Could you check a few things on this model? Use its own coordinates, in mm. A direction names the side the tool comes from. Round coordinates to 2 decimals unless told otherwise and drop trailing zeros. Loops run counter-clockwise (first coordinate to the right, second up) from the corner with the lowest first, then second, coordinate; pieces in that order, holes last. Notation, with made-up numbers: (48.25, -24.75) -> (100.25, -24.75) arc R24 ccw to (100.25, -11.75) -> close; hole circle Ø5 at (62, -23.5). An arc over 180 degrees is marked (long way). One line per item, written item: value.
Autodesk Inventor part; units mm, degrees
ref_plane "РабПлоскость1" through (0, 14.5, 0) normal (0, 1, 0) x (-1, 0, 0)
ref_plane "РабПлоскость2" through (0, 0, 18.5) normal (0, 0, 1) x (1, 0, 0)
ref_plane "YZ Plane" through (0, 0, 0) normal (1, 0, 0) x (0, 1, 0)
sketch "Эскиз1" plane through (0, 0, 0) normal (0, 0, 1) x (1, 0, 0)
  line L0 (0, 0) -> (-160, 0)
  line L1 (0, 0) -> (0, 15.4226)
  line L2 (0, 15.4226) -> (-1, 16)
  line L3 (-1, 16) -> (-60, 16)
  line L4 (-60, 16) -> (-60, 17.5)
  line L5 (-60, 17.5) -> (-80, 17.5)
  line L6 (-80, 17.5) -> (-80, 20)
  line L7 (-80, 20) -> (-140, 20)
  line L8 (-140, 20) -> (-140, 17.5)
  line L9 (-140, 17.5) -> (-160, 17.5)
  line L10 (-160, 17.5) -> (-160, 0)
  dimension "d0" = 160
  dimension "d1" = 32
  dimension "d2" = 30
  dimension "d3" = 1
  dimension "d4" = 60
  dimension "d5" = 35
  dimension "d6" = 20
  dimension "d7" = 40
revolve "Вращение1" add sketch "Эскиз1" angle 360 about axis through (0, 0, 0) along (-1, 0, 0)
ref_plane "РабПлоскость1" through (0, 14.5, 0) normal (0, 1, 0) x (-1, 0, 0)
ref_plane "РабПлоскость2" through (0, 0, 18.5) normal (0, 0, 1) x (1, 0, 0)
sketch "Эскиз3" plane through (0, 14.5, 0) normal (0, 1, 0) x (-1, 0, 0)
  line L0 (0, 15.4226) -> (0, -15.4226)
  line L1 (80, 20) -> (80, -20)
  line L2 (140, 20) -> (140, -20)
  line L3 (44, 0) -> (16, 0) construction
  line L4 (40, 4) -> (20, 4)
  line L5 (20, -4) -> (40, -4)
  arc A0 (40, -4) -> (40, 4) centre (40, 0) ccw
  arc A1 (20, 4) -> (20, -4) centre (20, 0) ccw
  point P0 (0, 0)
  point P1 (30, 0)
  point P2 (80, 0)
  dimension "d11" = 20
  dimension "d12" = 8
  dimension "d13" = 50
extrude "Выдавливание1" cut sketch "Эскиз3" along normal through all
sketch "Эскиз4" plane through (0, 0, 18.5) normal (0, 0, 1) x (1, 0, 0)
  line L0 (-124, 0) -> (-96, 0) construction
  line L1 (-120, -4) -> (-100, -4)
  line L2 (-100, 4) -> (-120, 4)
  arc A0 (-120, 4) -> (-120, -4) centre (-120, 0) ccw
  arc A1 (-100, -4) -> (-100, 4) centre (-100, 0) ccw
  line L3 (-80, -17.5) -> (-80, 17.5)
  point P0 (0, 0)
  point P1 (-110, 0)
  point P2 (-80, 0)
  dimension "d16" = 20
  dimension "d17" = 8
  dimension "d18" = 30
extrude "Выдавливание2" cut sketch "Эскиз4" along normal through all
properties part number "Shaft1"
Item 1: For faces 1 (the face through (-30.91, -3.47, 15.62)), 2 (the face through (-16, 15, 0)), 3 (the face through (-110, 0, 18.5)), 4 (the face through (-140, 0, 18)), which set-ups out of +Z, -Z, +X, -X, +Y, -Y let a thin tool reach every point of the face, with its end or its side?
Output:
face 1: +X
face 2: +Y
face 3: +Z
face 4: -X
Item 2: If we section it at A-A on z = 0: List the corners of the cut face in (x, y) for me, plus the area to 3 significant figures.
Output:
outline: (-160, -17.5) -> (-140, -17.5) -> (-140, -20) -> (-80, -20) -> (-80, -17.5) -> (-60, -17.5) -> (-60, -16) -> (-1, -16) -> (0, -15.42) -> (0, 15.42) -> (-1, 16) -> (-16, 16) -> (-16, 14.5) -> (-44, 14.5) -> (-44, 16) -> (-60, 16) -> (-60, 17.5) -> (-80, 17.5) -> (-80, 20) -> (-140, 20) -> (-140, 17.5) -> (-160, 17.5) -> close
area: 5,680 mm²
Item 3: If we section it at C-C on x = -14.5: List the corners of the cut face in (y, z) for me, plus the area to 3 significant figures.
Output:
outline: circle Ø32 at (0, 0)
area: 804 mm²
Item 4: Will these pins go through, and if not, where does the flat tip stop? pin 1 Ø2.5 at (x, z) = (-34, -0.5) entering from +Y; pin 2 Ø1 at (x, z) = (-39, -14.5) entering from -Y; pin 3 Ø3 at (x, z) = (-22.5, 15.5) entering from +Y.
Output:
pin 1: stops at y = 14.5
pin 2: stops at y = -7.75
pin 3: stops at y = 7.75
Item 5: If we mould it in two halves opening along Y, with no side actions, what happens to faces 5 (the face through (-96, 0, 19)), 6 (the face through (-30, 14.5, 0)), 7 (the face through (-110.42, -4.336, 19.524)), 8 (the face through (0, 0, 0))? For each: released by +Y, released by -Y, zero draft, split by the parting line, or undercut.
Output:
face 5: undercut
face 6: released by +Y
face 7: split by the parting line
face 8: zero draft
Item 6: I need wall thicknesses on line 1 (X direction, y = 11.5, z = 13.5); line 2 (X direction, y = -8, z = -14); line 3 (Y direction, x = -84, z = 1). Which ranges of each line are inside material? Lowest first, please. Write a range as from..to.
Output:
line 1: x = -140..-80
line 2: x = -160..-60
line 3: y = -19.97..19.97
Item 7: If we section it at B-B on y = 0: List the corners of the cut face in (x, z) for me, plus the area to 3 significant figures.
Output:
outline: (-160, -17.5) -> (-140, -17.5) -> (-140, -20) -> (-80, -20) -> (-80, -17.5) -> (-60, -17.5) -> (-60, -16) -> (-1, -16) -> (0, -15.42) -> (0, 15.42) -> (-1, 16) -> (-60, 16) -> (-60, 17.5) -> (-80, 17.5) -> (-80, 20) -> (-96, 20) -> (-96, 18.5) -> (-124, 18.5) -> (-124, 20) -> (-140, 20) -> (-140, 17.5) -> (-160, 17.5) -> close
area: 5,680 mm²
Item 8: If we section it at D-D on x = -62.5: List the corners of the cut face in (y, z) for me, plus the area to 3 significant figures.
Output:
outline: circle Ø35 at (0, 0)
area: 962 mm²
